Autodesk Fusion 360 part; units mm, degrees
sketch "Sketch1" plane through (0, 0, 0) normal (0, 1, 0) x (1, 0, 0)
  line L0 (-36.25, -23.375) -> (36.25, -23.375)
  line L1 (36.25, -23.375) -> (36.25, 23.375)
  line L2 (36.25, 23.375) -> (-36.25, 23.375)
  line L3 (-36.25, 23.375) -> (-36.25, -23.375)
  dimension "d62" = 72.5
  dimension "d63" = 46.75
  dimension "d64" = 23.375
  dimension "d65" = 36.25
extrude "Extrude9" add sketch "Sketch1" along normal blind 60
sketch "Sketch8" plane through (0, 0, 0) normal (0, 1, 0) x (1, 0, 0)
  line L0 (-5, -4.625) -> (5, -4.625)
  line L1 (-5, 18.375) -> (5, 18.375)
  arc A0 (-5, 18.375) -> (-5, -4.625) centre (-5, 6.875) ccw
  arc A1 (5, -4.625) -> (5, 18.375) centre (5, 6.875) ccw
  line L2 (36.25, 23.375) -> (-36.25, 23.375)
  line L3 (36.25, 23.375) -> (-36.25, 23.375)
  dimension "d39" = 10
  dimension "d40" = 5
  dimension "d94" = 23
  dimension "d123" = 28
extrude "Extrude10" cut sketch "Sketch8" along normal blind 95
sketch "Sketch9" plane through (0, 0, -23.375) normal (0, 0, -1) x (1, 0, 0)
  line L0 (36.25, 0) -> (-36.25, 0)
  line L1 (-36.25, 0) -> (-36.25, -60)
  line L2 (-36.25, -60) -> (36.25, -60)
  line L3 (36.25, -60) -> (36.25, 0)
  line L4 (-5, -33) -> (5, -33)
  line L5 (-5, -58) -> (5, -58)
  arc A0 (-5, -33) -> (-5, -58) centre (-5, -45.5) ccw
  arc A1 (5, -58) -> (5, -33) centre (5, -45.5) ccw
  dimension "d45" = 10
  dimension "d46" = 10
  dimension "d47" = 5
  dimension "d75" = 2
  dimension "d95" = 25
extrude "Extrude11" cut sketch "Sketch9" against normal blind 12 contours L4 L5 A0 A1
sketch "Sketch10" plane through (0, 60, 0) normal (0, 1, 0) x (-1, 0, 0)
  line L0 (36.25, -23.375) -> (36.25, 23.375)
  line L1 (36.25, 23.375) -> (-36.25, 23.375)
  line L2 (-36.25, 23.375) -> (-36.25, -23.375)
  line L3 (-36.25, -23.375) -> (36.25, -23.375)
  line L4 (-67.5, 27.5) -> (67.5, 27.5)
  line L5 (67.5, 27.5) -> (67.5, -27.5)
  line L6 (67.5, -27.5) -> (-67.5, -27.5)
  line L7 (-67.5, -27.5) -> (-67.5, 27.5)
  line L8 (5, -18.375) -> (-5, -18.375)
  arc A0 (-5, 4.625) -> (-5, -18.375) centre (-5, -6.875) ccw
  line L9 (-5, 4.625) -> (5, 4.625)
  arc A1 (5, -18.375) -> (5, 4.625) centre (5, -6.875) ccw
  line L10 (57.5, -6.5) -> (57.5, -24.5)
  line L11 (57.5, -24.5) -> (-57.5, -24.5)
  line L12 (-57.5, -24.5) -> (-57.5, -1.5)
  line L13 (-57.5, -1.5) -> (-44.5, -1.5)
  line L14 (-44.5, -1.5) -> (-44.5, -6.5)
  line L15 (-57.5, -12.4536) -> (-57.5, -1.5)
  line L16 (-44.5, -6.5) -> (57.5, -6.5)
  dimension "d50" = 135
  dimension "d51" = 55
  dimension "d52" = 27.5
  dimension "d53" = 67.5
  dimension "d141" = 115
  dimension "d142" = 10
  dimension "d143" = 13
  dimension "d144" = 23
  dimension "d145" = 18
  dimension "d146" = 3
extrude "Extrude12" add sketch "Sketch10" along normal blind 5.5 contours L0 L2 L3 L8 A0 A1 L16 | L0 L2 L3 L10 L11 L12 L13 L14 L15 L16 | L0 L1 L2 A0 L9 A1 L16 | A0 L9 A1 L16 | L8 A0 A1 L16 | L4 L5 L6 L7
sketch "Sketch13" plane through (0, 0, -23.375) normal (0, 0, -1) x (1, 0, 0)
  line L0 (5, -58) -> (-5, -58)
  arc A0 (-5, -33) -> (-5, -58) centre (-5, -45.5) ccw
  line L1 (-5, -33) -> (5, -33)
  arc A1 (5, -58) -> (5, -33) centre (5, -45.5) ccw
  line L2 (36.25, 0) -> (-36.25, 0)
  line L3 (-36.25, 0) -> (-36.25, -60)
  line L4 (-36.25, -60) -> (36.25, -60)
  line L5 (36.25, -60) -> (36.25, 0)
  line L6 (-36.25, -30.2113) -> (36.25, -30.2113)
  line L7 (36.25, -30.2113) -> (36.25, -25)
  line L8 (36.25, -25) -> (-36.25, -25)
  line L9 (-36.25, -25) -> (-36.25, -30.2113)
  dimension "d113" = 25
extrude "Extrude17" add sketch "Sketch13" along normal blind 2 contours L3 L5 L6 L7 L8 L9
sketch "Sketch14" plane through (0, 65.5, 0) normal (0, 1, 0) x (-1, 0, 0)
  line L0 (-67.5, -27.5) -> (67.5, -27.5)
  line L1 (67.5, -27.5) -> (67.5, 27.5)
  line L2 (67.5, 27.5) -> (-67.5, 27.5)
  line L3 (-67.5, 27.5) -> (-67.5, -27.5)
  circle A0 centre (-62.5, 22.5) radius 2
  circle A1 centre (-62.5, -22.5) radius 2
  circle A2 centre (62.5, 22.5) radius 2
  circle A3 centre (62.5, -22.5) radius 2
  dimension "d78" = 4
  dimension "d79" = 4
  dimension "d80" = 4
  dimension "d81" = 4
  dimension "d83" = 5
  dimension "d84" = 5
  dimension "d85" = 5
  dimension "d86" = 5
  dimension "d88" = 5
  dimension "d89" = 5
  dimension "d90" = 5
  dimension "d91" = 5
extrude "Extrude18" cut sketch "Sketch14" against normal blind 15 contours A0 | A1 | A2 | A3
fillet "Fillet1" radius 2 2 edges at (0, 30.2113, -25.375) (0, 30.2113, -23.375)
sketch "Sketch15" plane through (0, 0, 0) normal (0, -1, 0) x (1, 0, 0)
  line L0 (5, -18.375) -> (-5, -18.375)
  arc A0 (-5, 4.625) -> (-5, -18.375) centre (-5, -6.875) ccw
  line L1 (-5, 4.625) -> (5, 4.625)
  arc A1 (5, -18.375) -> (5, 4.625) centre (5, -6.875) ccw
  line L2 (-36.25, 23.375) -> (-36.25, -23.375)
  line L3 (-36.25, -23.375) -> (36.25, -23.375)
  line L4 (36.25, -23.375) -> (36.25, 23.375)
  line L5 (36.25, 23.375) -> (-36.25, 23.375)
  circle A2 centre (-6, 11.5) radius 2
  circle A3 centre (6, 11.5) radius 2
  dimension "d99" = 4
  dimension "d100" = 4
  dimension "d101" = 12
  dimension "d102" = 6
  dimension "d103" = 6
  dimension "d140" = 11.5
extrude "Extrude19" cut sketch "Sketch15" against normal blind 20 contours A2 | A3
ref_plane "WorkPlane1" through (0, 30, 0) normal (0, 0, -1) x (-1, 0, 0)
mirror "Mirror2" about plane through (0, 30, 0) normal (0, 0, -1) of "Extrude17"
sketch "Sketch17" plane through (0, 0, 0) normal (0, -1, 0) x (1, 0, 0)
  line L0 (5, -18.375) -> (-5, -18.375)
  arc A0 (-5, 4.625) -> (-5, -18.375) centre (-5, -6.875) ccw
  line L1 (-5, 4.625) -> (5, 4.625)
  arc A1 (5, -18.375) -> (5, 4.625) centre (5, -6.875) ccw
  line L2 (-36.25, 23.375) -> (-36.25, -23.375)
  line L3 (-36.25, -23.375) -> (36.25, -23.375)
  line L4 (36.25, -23.375) -> (36.25, 23.375)
  line L5 (36.25, 23.375) -> (-36.25, 23.375)
  circle A2 centre (-5, -6.875) radius 3
  circle A3 centre (5, -6.875) radius 3
  line L6 (-5, 4.625) -> (5, 4.625)
  line L7 (-5, -18.375) -> (5, -18.375)
  circle A4 centre (-6, 11.5) radius 2
  circle A5 centre (6, 11.5) radius 2
  dimension "d114" = 6
fillet "Fillet3" radius 2.5 4 edges at (0, 60, 27.5) (-67.5, 60, 0) (67.5, 60, 0) (0, 60, -27.5)
fillet "Fillet7" radius 2 1 edges at (0, 30.2113, 23.375)
fillet "Fillet10" radius 10 2 edges at (36.25, 60, 0) (-36.25, 60, 0)
sketch "Sketch18" plane through (0, 0, 0) normal (0, -1, 0) x (1, 0, 0)
  circle A0 centre (-6, 11.5) radius 2
  circle A1 centre (6, 11.5) radius 2
  line L0 (5, -18.375) -> (-5, -18.375)
  arc A2 (-5, 4.625) -> (-5, -18.375) centre (-5, -6.875) ccw
  line L1 (-5, 4.625) -> (5, 4.625)
  arc A3 (5, -18.375) -> (5, 4.625) centre (5, -6.875) ccw
  line L2 (-36.25, 23.375) -> (-36.25, -23.375)
  line L3 (-36.25, -23.375) -> (36.25, -23.375)
  line L4 (36.25, -23.375) -> (36.25, 23.375)
  line L5 (36.25, 23.375) -> (-36.25, 23.375)
  line L6 (-33.75, -20.875) -> (33.75, -20.875)
  line L7 (33.75, -20.875) -> (33.75, 20.875)
  line L8 (33.75, 20.875) -> (-33.75, 20.875)
  line L9 (-33.75, 20.875) -> (-33.75, -20.875)
  dimension "d134" = -2.5
extrude "Extrude21" cut sketch "Sketch18" against normal blind 25 contours L2 L3 L4 L5
sketch "Sketch19" plane through (0, 0, 0) normal (0, -1, 0) x (1, 0, 0)
  line L0 (33.75, 20.875) -> (-33.75, 20.875)
  line L1 (-33.75, 20.875) -> (-33.75, -20.875)
  line L2 (-33.75, -20.875) -> (33.75, -20.875)
  line L3 (33.75, -20.875) -> (33.75, 20.875)
  circle A0 centre (-6, 11.5) radius 2
  circle A1 centre (6, 11.5) radius 2
  line L4 (5, -18.375) -> (-5, -18.375)
  arc A2 (-5, 4.625) -> (-5, -18.375) centre (-5, -6.875) ccw
  line L5 (-5, 4.625) -> (5, 4.625)
  arc A3 (5, -18.375) -> (5, 4.625) centre (5, -6.875) ccw
  line L6 (-32.4071, 0) -> (-31.9234, 9.9156) construction
  line L7 (-31.9234, 9.9156) -> (-18.8638, 18.622) construction
  line L8 (-18.8638, 18.622) -> (-5.8043, 20.875) construction
  line L9 (-5.8043, 20.875) -> (0, 20.875) construction
  spline S0 degree 4 poles (-32.4071, 0) (-31.9234, 9.9156) (-18.8638, 18.622) (-5.8043, 20.875) (0, 20.875) knots 0 0 0 0 0 1 1 1 1 1
  line L10 (-78.035, 0) -> (72.5532, 0) construction
  line L11 (0, 0) -> (0, 55.866) construction
  spline S1 degree 4 poles (32.4071, 0) (31.9234, 9.9156) (18.8638, 18.622) (5.8043, 20.875) (0, 20.875) knots 0 0 0 0 0 1 1 1 1 1
  line L12 (32.4071, 0) -> (31.9234, 9.9156) construction
  line L13 (31.9234, 9.9156) -> (18.8638, 18.622) construction
  line L14 (18.8638, 18.622) -> (5.8043, 20.875) construction
  line L15 (5.8043, 20.875) -> (0, 20.875) construction
  spline S2 degree 4 poles (-32.4071, 0) (-31.9234, -9.9156) (-18.8638, -18.622) (-5.8043, -20.875) (0, -20.875) knots 0 0 0 0 0 1 1 1 1 1
  line L16 (-32.4071, 0) -> (-31.9234, -9.9156) construction
  line L17 (-31.9234, -9.9156) -> (-18.8638, -18.622) construction
  line L18 (-18.8638, -18.622) -> (-5.8043, -20.875) construction
  line L19 (-5.8043, -20.875) -> (0, -20.875) construction
  spline S3 degree 4 poles (32.4071, 0) (31.9234, -9.9156) (18.8638, -18.622) (5.8043, -20.875) (0, -20.875) knots 0 0 0 0 0 1 1 1 1 1
  line L20 (32.4071, 0) -> (31.9234, -9.9156) construction
  line L21 (31.9234, -9.9156) -> (18.8638, -18.622) construction
  line L22 (18.8638, -18.622) -> (5.8043, -20.875) construction
  line L23 (5.8043, -20.875) -> (0, -20.875) construction
extrude "Extrude22" cut sketch "Sketch19" against normal blind 25 contours L0 L2 L3 S1 S3 | L0 L1 L2 S0 S2
sketch "Sketch20" plane through (0, 65.5, 0) normal (0, 1, 0) x (-1, 0, 0)
  line L0 (-44.5, -6.5) -> (57.5, -6.5)
  line L1 (-44.5, -1.5) -> (-44.5, -6.5)
  line L2 (-57.5, -1.5) -> (-44.5, -1.5)
  line L3 (57.5, -6.5) -> (57.5, -24.5)
  line L4 (-57.5, -24.5) -> (-57.5, -1.5)
  line L5 (57.5, -24.5) -> (-57.5, -24.5)
  line L6 (-57.5, -12.4536) -> (-57.5, -1.5)
  line L7 (-67.5, -27.5) -> (-67.5, 27.5)
  line L8 (67.5, -27.5) -> (-67.5, -27.5)
  dimension "d147" = 115
  dimension "d148" = 13
  dimension "d149" = 23
  dimension "d150" = 18
  dimension "d151" = 10
  dimension "d152" = 3
extrude "Extrude23" cut sketch "Sketch20" against normal blind 3.5
equation "d52 = ( 55 / 2 ) * 1 mm"
equation "d53 = ( 135 / 2 ) * 1 mm"
equation "d64 = ( 46.75 / 2 ) * 1 mm"
equation "d65 = ( 72.5 / 2 ) * 1 mm"
equation "d108 = -( ( 46.75 / 2 ) * 1 mm )"
Work out the finished part from the listing and answer in its coordinate system (mm). A direction names the side the tool comes from. Give positions to 0.01 mm unless a question says otherwise; leave off trailing zeros. Write each loop counter-clockwise with the first axis right and the second up, starting at its lowest first coordinate (ties: lowest second). Pieces come first, ordered by that corner, then holes. Notation, with made-up numbers: (82, 11) -> (124, 11) arc R18 cw to (124, 32) -> close; hole circle Ø3 at (7.25, -20.75). An arc over 180 degrees is marked (long way). Write each question's results on one line, items separated by ' | '.
1. A tool of negligible diameter and unlimited length cuts with its end or side. For faces 1 (the cylindrical face through (62.76, 62.788, -20.517)), 2 (the flat face through (-1, 27, -25.375)), 3 (the cylindrical face through (-17.497, 45.225, -18.792)), 4 (the flat face through (-1, 64, -27.5)), 5 (the flat face through (6, 20, 12)), from which of +Z, -Z, +X, -X, +Y, -Y can it reach the whole face along a straight path? Write none if from no direction.
Data:
face 1: +Y, -Y | face 2: -Z, +X, -X, -Y | face 3: -Z | face 4: -Z, +X, -X, +Y, -Y | face 5: -Y
2. Determine the mould class of faces 6 (the flat face through (44.5, 64, -4)), 7 (the cylindrical face through (-39.1, 56.99, 0.33)), 8 (the flat face through (-1, 46, 23.375)), 9 (the flat face through (0, 58, -21)) for opening direction X: +X half, -X half, draft (parallel to the pull), parting line (faces both ways), or undercut.
Data:
face 6: undercut | face 7: -X half | face 8: draft | face 9: undercut
3. Find section A-A on x = 62.5. Determine the outline of the cut face in (y, z), and give its area (3 significant figures).
Data:
outline: (60, -25) arc R2.5 ccw to (62.5, -27.5) -> (65.5, -27.5) -> (65.5, -24.5) -> (60, -24.5) -> close; (60, -20.5) -> (65.5, -20.5) -> (65.5, 20.5) -> (60, 20.5) -> close; (60, 24.5) -> (65.5, 24.5) -> (65.5, 27.5) -> (62.5, 27.5) arc R2.5 ccw to (60, 25) -> close | area: 256 mm^2
4. Each of these flat-tipped pins is pushed along its axis until it touches: pin 1 Ø12 at (x, y) = (-37, 49.5) entering from -Z (3 decimals); pin 2 Ø6 at (x, y) = (8.5, 9.5) entering from +Z; pin 3 Ø1.5 at (y, z) = (15.5, -1) entering from +X. Where does it stop, or does it pass through?
Data:
pin 1: z = -23.375 | pin 2: z = 20.33 | pin 3: x = 32.39
5. Find section C-C on x = 48.5. Determine the outline of the cut face in (y, z), and give its area (3 significant figures).
Data:
outline: (60, -25) arc R2.5 ccw to (62.5, -27.5) -> (65.5, -27.5) -> (65.5, -24.5) -> (62, -24.5) -> (62, -1.5) -> (65.5, -1.5) -> (65.5, 27.5) -> (62.5, 27.5) arc R2.5 ccw to (60, 25) -> close | area: 219 mm^2
6. Straight lines are drawn through the part: L1, parallel to Z at x = -62.5, y = 62.7; L2, parallel to Z at x = -62, y = 64; L3, parallel to Y at x = 48.5, z = 12.5. For each, find the intervals that lie inside material, in ascending order.
Data:
L1: -27.5 to -24.5, -20.5 to 20.5, 24.5 to 27.5 | L2: -27.5 to -24.44, -20.56 to 20.56, 24.44 to 27.5 | L3: 60 to 65.5
7. Find section D-D on y = 12. Give the number of separate pieces and of enclosed holes in the cut face, and give its area (3 significant figures).
Data:
separate pieces: 1 | enclosed holes: 3 | area: 1,350 mm^2
8. Find section B-B on y = 42. Determine the outline of the cut face in (x, z) (3 decimals), and give its area (3 significant figures).
Data:
outline: (-36.25, -23.375) -> (-17, -23.375) -> (-17, -11.375) -> (-15.583, -11.375) arc R11.5 cw to (-5, 4.625) -> (5, 4.625) arc R11.5 cw to (15.583, -11.375) -> (17, -11.375) -> (17, -23.375) -> (36.25, -23.375) -> (36.25, 23.375) -> (-36.25, 23.375) -> close | area: 2,510 mm^2
